Can you work these out from the model? Positions are in its coordinate system, mm. A direction names the side the tool comes from. Round coordinates to 2 decimals unless told otherwise and drop trailing zeros. Write each loop counter-clockwise with the first axis right and the second up, starting at its lowest first coordinate (ties: lowest second). Pieces come first, ordered by that corner, then holes. Notation, with made-up numbers: M 50,6.5 L 77,6.5 A24 ccw 77,34.5 Z; hole C 15,77.5 d9. An arc over 180 degrees is marked long. Answer in a Markdown table with one row per item. Add a question column.
(1) If we mould it in two halves opening along Z, with no side actions, what happens to faces 1 (the face through (-3.21, 0.9, -2.86)), 2 (the face through (0, -2, 0)), 3 (the face through (-3.3, -0.05, 1.23))? For each: released by +Z, released by -Z, zero draft, split by the parting line, or undercut.
(2) Suppose I cut it at B-B, the plane x = -0.5. Write out the boundary of the cut face in (y, z), then the cut area to 3 significant figures.
(3) Suppose I cut it at A-A, the plane z = 0. Write out the boundary of the cut face in (x, y).
(4) I'm going to push flat-ended pins straight in: pin 1 (0.5 mm diameter, centred on x = -0.5, z = 2, fed in from +Y); pin 2 (1.1 mm diameter, centred on x = -0.5, z = -2, fed in from +Y); pin 3 (0.5 mm diameter, centred on y = 0, z = -2.5, fed in from +X). Where does each tip first touch, or does it pass through?
(5) If I drill on probe 1 along Y at (x, z) = (-5.5, 0.5); probe 2 along Y at (x, z) = (-2.75, 0), over which ranges is the centre line in solid material (lowest first)?
(6) Suppose I cut it at C-C, the plane x = -1.25. Write out the boundary of the cut face in (y, z).
(7) For faces 4 (the face through (0, 2, 0)), 5 (the face through (-0.5, 0.5, -2.1)), which set-ups out of +Z, -Z, +X, -X, +Y, -Y let a thin tool reach every point of the face, with its end or its side?
Autodesk Inventor part; units mm, degrees
ref_plane "YZ Plane" through (0, 0, 0) normal (1, 0, 0) x (0, 1, 0)
ref_plane "XZ Plane" through (0, 0, 0) normal (0, 1, 0) x (-1, 0, 0)
ref_plane "XY Plane" through (0, 0, 0) normal (0, 0, 1) x (1, 0, 0)
sketch "スケッチ1" plane through (0, 0, 0) normal (0, 1, 0) x (-1, 0, 0)
  line L0 (0, 0) -> (6.5, 0)
  line L1 (6.5, 0) -> (6.5, -3)
  line L2 (6.5, -3) -> (0, -3)
  line L3 (0, -3) -> (0, 0)
  dimension "d0" = 6.5
  dimension "d1" = 3
revolve "回転1" add sketch "スケッチ1" angle 360 about axis through (0, 0, 0) along (-1, 0, 0)
sketch "スケッチ2" plane through (0, 0, 0) normal (1, 0, 0) x (0, 0, -1)
  point P0 (0, 0)
  point P1 (0, 0)
hole "穴1" at (0, 0, 0) direction (-1, 0, 0) diameter 2.459 end through all
sketch "スケッチ3" plane through (0, 0, 0) normal (1, 0, 0) x (0, 0, -1)
  circle A0 centre (0, 0) radius 3
  line L0 (3, 0) -> (-3, 0)
  line L1 (3, -0.5) -> (-3, -0.5)
  line L2 (3, 0.5) -> (-3, 0.5)
  line L3 (3, 0.5) -> (3, -0.5)
  line L4 (-3, 0.5) -> (-3, -0.5)
  point P0 (-2.958, -0.5)
  point P1 (2.958, -0.5)
  point P2 (2.958, 0.5)
  point P3 (-2.958, 0.5)
  dimension "d10" = 0.5
extrude "押し出し1" cut sketch "スケッチ3" against normal blind 1 contours L0 A0 L2 | A0 L1 L0
chamfer "面取り1" distance 0.3 angle 45 3 edges at (-6.5, 0, 3) (0, 3, 0) (0, -3, 0)
properties part number "ARU-306_5SMO" material "ステンレス鋼 AISI 304"
Calculated:
| question | item | result |
|---|---|---|
| 1 | face 1 | split by the parting line |
| 1 | face 2 | zero draft |
| 1 | face 3 | undercut |
| 2 | outline | M -0.5,-2.96 L -0.5,-1.12 A1.23 cw -0.5,1.12 L -0.5,2.96 A3 ccw Z; M 0.5,-2.96 A3 ccw 0.5,2.96 L 0.5,1.12 A1.23 cw 0.5,-1.12 Z |
| 2 | area | 19.9 mm² |
| 3 | outline | M -6.5,-2.7 L -6.2,-3 L -0.3,-3 L 0,-2.7 L 0,-1.23 L -6.5,-1.23 Z; M -6.5,1.23 L 0,1.23 L 0,2.7 L -0.3,3 L -6.2,3 L -6.5,2.7 Z |
| 4 | pin 1 | y = 2.44 |
| 4 | pin 2 | y = 2.63 |
| 4 | pin 3 | x = -1 |
| 5 | probe 1 | -2.96 to -1.12, 1.12 to 2.96 |
| 5 | probe 2 | -3 to -1.23, 1.23 to 3 |
| 6 | outline | C 0,0 d6; hole C 0,0 d2.46 |
| 7 | face 4 | +Z, -Z, +X, +Y, -Y |
| 7 | face 5 | +Z, -Z, +X |
